Geometry check sheet. Reference: drawing and pictorial views, mm from the part's lowest x, y, z. A direction names the side the tool comes from. Round coordinates to 2 decimals unless told otherwise and drop trailing zeros. Write each loop counter-clockwise with the first axis right and the second up, starting at its lowest first coordinate (ties: lowest second). Pieces come first, ordered by that corner, then holes. Notation, with made-up numbers: (82.5, 69.5) -> (127.5, 69.5) arc R26 ccw to (127.5, 88.5) -> close; hole circle Ø11 at (57, 89.5). An arc over 180 degrees is marked (long way). Write item = value, one per line.
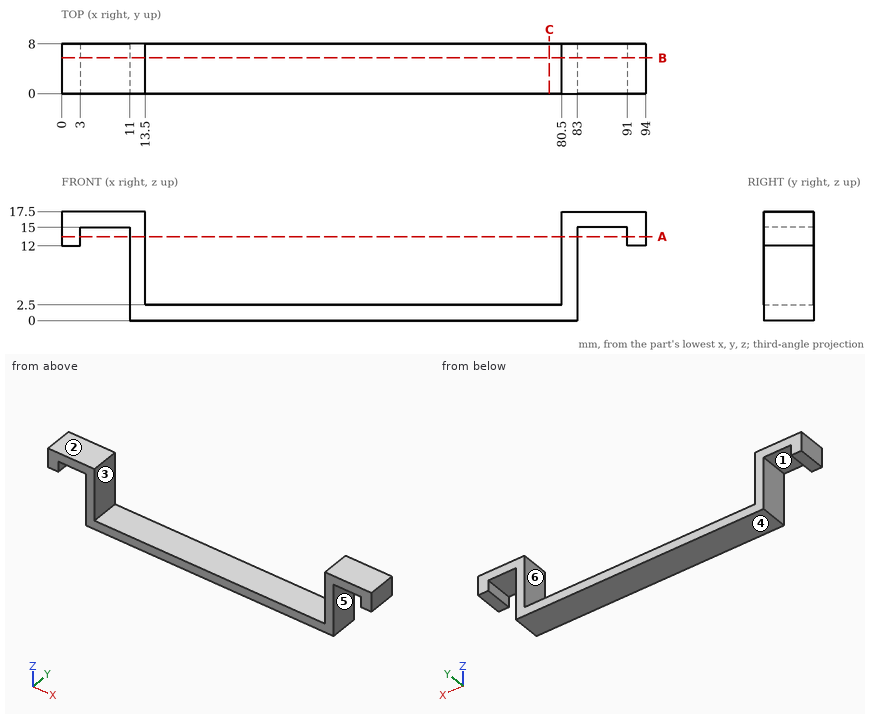
(1) Go/stop test with flat-tipped pins: P1, Ø1.5, axis at y = 4.5, z = 14, coming from the -X side; P2, Ø1.5, axis at y = 5, z = 8, coming from the -X side; P3, Ø2, axis at x = 25.5, y = 7, coming from the +Z side; P4, Ø4, axis at x = 87, y = 3, coming from the -Z side. Record where each tip stops, or that it passes through.
Worked answers:
P1 = 0
P2 = 11
P3 = 2.5
P4 = 15
(2) Sectioned sample at B-B on y = 5.75. Enter the section's corners in (x, z), then the cut area to 3 significant figures.
Worked answers:
outline = (0, 12) -> (3, 12) -> (3, 15) -> (11, 15) -> (11, 0) -> (83, 0) -> (83, 15) -> (91, 15) -> (91, 12) -> (94, 12) -> (94, 17.5) -> (80.5, 17.5) -> (80.5, 2.5) -> (13.5, 2.5) -> (13.5, 17.5) -> (0, 17.5) -> close
area = 328 mm²
(3) Material ranges on L1, parallel to X at y = 3, z = 2.75; L2, parallel to X at y = 4.5, z = 16.75; L3, parallel to Z at x = 43.5, y = 1.75, recorded low to high. Write a range as [from, to].
Worked answers:
L1 = [11, 13.5], [80.5, 83]
L2 = [0, 13.5], [80.5, 94]
L3 = [0, 2.5]
(4) Access from +Z, -Z, +X, -X, +Y, -Y to the whole of each face (thin tool, end or side, straight path). Record for the marked faces 4, 5 and 6.
Worked answers:
face_4 = -Z, +X, -X, +Y, -Y
face_5 = -Z, +Y, -Y
face_6 = +Z, +Y, -Y
(5) Sectioned sample at A-A on z = 13.5. Enter the section's corners in (x, y), then the cut area to 3 significant figures.
Worked answers:
outline = (0, 0) -> (3, 0) -> (3, 8) -> (0, 8) -> close; (11, 0) -> (13.5, 0) -> (13.5, 8) -> (11, 8) -> close; (80.5, 0) -> (83, 0) -> (83, 8) -> (80.5, 8) -> close; (91, 0) -> (94, 0) -> (94, 8) -> (91, 8) -> close
area = 88.0 mm²
(6) Release check for a two-part mould opening along X. For the marked faces 1, 2 and 3 record: pulls with the +X half, pulls with the -X half, needs draft (parallel to the pull), parting line crosses it, or undercut.
Worked answers:
face_1 = undercut
face_2 = needs draft
face_3 = undercut
(7) Sectioned sample at C-C on x = 78.5. Enter the section's corners in (y, z), then the cut area to 3 significant figures.
Worked answers:
outline = (0, 0) -> (8, 0) -> (8, 2.5) -> (0, 2.5) -> close
area = 20.0 mm²
